from build123d import *

# Parameters (mm, degrees)
SKETCH1_R            = 17.78
SKETCH1_R_2          = 0.762
BOSS_EXTRUDE1_DEPTH  = 5
SKETCH5_R            = 2.667
CUT_EXTRUDE1_DEPTH   = 3
M5_CLEARANCE_HOLE2_D = 5.8


with BuildPart() as part:
    # Sketch1 → Boss-Extrude1 (new body)
    with BuildSketch(Plane(origin=(0, 0, 0), x_dir=(1, 0, 0), z_dir=(0, 1, 0))):
        with Locations(Location((0, 0, 0), (0, 0, 270))):
            Circle(SKETCH1_R)
        with Locations(Location((-14.478, 0, 0), (0, 0, 270))):
            Circle(SKETCH1_R_2, mode=Mode.SUBTRACT)
        with Locations(Location((14.478, 0, 0), (0, 0, 270))):
            Circle(SKETCH1_R_2, mode=Mode.SUBTRACT)
    extrude(amount=BOSS_EXTRUDE1_DEPTH)

    # Sketch5 → Cut-Extrude1 (cut)
    with BuildSketch(Plane.XZ):
        with Locations(Location((0, 13.97, 0), (0, 0, 270))):
            Circle(SKETCH5_R)
    extrude(amount=-CUT_EXTRUDE1_DEPTH, mode=Mode.SUBTRACT)

    # M5 Clearance Hole2 (through all)
    with Locations(Plane(origin=(0, 5, 0), x_dir=(1, 0, 0), z_dir=(0, 1, 0))):
        with Locations((0, 0)):
            Hole(M5_CLEARANCE_HOLE2_D / 2)


solid = part.part
Geometry check sheet. Reference: the model listing, model coordinates, mm. A direction names the side the tool comes from. Give positions to 0.01 mm unless a question says otherwise; leave off trailing zeros. Write each loop counter-clockwise with the first axis right and the second up, starting at its lowest first coordinate (ties: lowest second). Pieces come first, ordered by that corner, then holes. Notation, with made-up numbers: (-24.5, 22.25) - (30.5, 22.25) arc R23 ccw to (30.5, 30.25) - close; hole circle Ø4 at (11, 23). An arc over 180 degrees is marked (long way). Put each result on its own line as item: value.
1. Sectioned sample at D-D, the plane z = 13.97. Enter the section's corners in (x, y), plus the area to 3 significant figures.
Ans:
outline: (-11, 0) - (-2.67, 0) - (-2.67, 3) - (2.67, 3) - (2.67, 0) - (11, 0) - (11, 5) - (-11, 5) - close
area: 94.0 mm²
2. Go/stop test with flat-tipped pins: pin 1 (0.9 mm diameter, centred on x = 14.478, z = 0, fed in from -Y); pin 2 (1 mm diameter, centred on x = -12.5, y = 3, fed in from -Z); pin 3 (1.6 mm diameter, centred on x = 1.5, z = 15, fed in from -Y); pin 4 (3 mm diameter, centred on x = 11.5, y = 2.5, fed in from -Z). Record where each tip stops, or that it passes through.
Ans:
pin 1: passes through
pin 2: stops at z = -13.12
pin 3: stops at y = 3
pin 4: stops at z = -14.7
3. Set-up check for faces 4 (the cylindrical face through (13.734, 2.465, -0.165)), 5 (the cylindrical face through (-1.62, 1.48, 16.09)): record each of +Z, -Z, +X, -X, +Y, -Y from which the full face is reachable in a straight line by a thin tool's end or side.
Ans:
face 4: +Y, -Y
face 5: -Y
4. Thickness scan on line 1 (Z direction, x = 0.5, y = 3.85); line 2 (Z direction, x = 14, y = 3.55); line 3 (Z direction, x = -11, y = 0.4). Record the ranges inside material, lowest first.
Ans:
line 1: z = -17.77 to -2.86, 2.86 to 17.77
line 2: z = -10.96 to -0.59, 0.59 to 10.96
line 3: z = -13.97 to 13.97
5. Sectioned sample at A-A, the plane z = 0. Enter the section's corners in (x, y).
Ans:
outline: (-17.78, 0) - (-15.24, 0) - (-15.24, 5) - (-17.78, 5) - close; (-13.72, 0) - (-2.9, 0) - (-2.9, 5) - (-13.72, 5) - close; (2.9, 0) - (13.72, 0) - (13.72, 5) - (2.9, 5) - close; (15.24, 0) - (17.78, 0) - (17.78, 5) - (15.24, 5) - close
6. Draft check along Z on faces 1 (the cylindrical face through (-17.36, 2.46, -3.85)), 2 (the flat face through (-4, 5, 0)), 3 (the cylindrical face through (-13.722, 2.465, -0.099)). Enter one of: +Z half, -Z half, draft (parallel to the pull), parting line (faces both ways), or undercut.
Ans:
face 1: parting line
face 2: draft
face 3: undercut
7. Sectioned sample at C-C, the plane y = 1.45. Enter the section's corners in (x, z), plus the area to 3 significant figures.
Ans:
outline: circle Ø35.56 at (0, 0); hole circle Ø1.52 at (-14.48, 0); hole circle Ø5.8 at (0, 0); hole circle Ø5.33 at (0, 13.97); hole circle Ø1.52 at (14.48, 0)
area: 941 mm²
8. Sectioned sample at B-B, the plane x = 0. Enter the section's corners in (y, z).
Ans:
outline: (0, -17.78) - (5, -17.78) - (5, -2.9) - (0, -2.9) - close; (0, 2.9) - (5, 2.9) - (5, 17.78) - (0, 17.78) - (0, 16.64) - (3, 16.64) - (3, 11.3) - (0, 11.3) - close
